Build history of the part. All positions in model axes, mm. A direction names the side the tool comes from. Round coordinates to 2 decimals unless told otherwise and drop trailing zeros. Loops run counter-clockwise (first coordinate to the right, second up) from the corner with the lowest first, then second, coordinate; pieces in that order, holes last. Notation, with made-up numbers: (54.25, -37.5) - (90.25, -37.5) arc R20 cw to (90.25, -16.5) - close; hole circle Ø11 at (72, 63.5). An arc over 180 degrees is marked (long way). Put each result on its own line as item: value. Start each with the question number.
from build123d import *

# Parameters (mm, degrees)
SKETCH1_W           = 10
SKETCH1_H           = 5
BOSS_EXTRUDE1_DEPTH = 5
SKETCH2_R           = 2.5
BOSS_EXTRUDE2_DEPTH = 5


with BuildPart() as part:
    # Sketch1 → Boss-Extrude1 (new body)
    with BuildSketch(Plane.XY):
        with Locations((-5, 2.5)):
            Rectangle(SKETCH1_W, SKETCH1_H)
    extrude(amount=BOSS_EXTRUDE1_DEPTH)

    # Sketch2 → Boss-Extrude2 (add)
    with BuildSketch(Plane.XY.offset(5)):
        with Locations(Location((-5, 2.5, 0), (0, 0, 270))):
            Circle(SKETCH2_R)
    extrude(amount=BOSS_EXTRUDE2_DEPTH)


solid = part.part
Item 1: Slice it at A-A (y = 2.5). Give the cut face in (x, z).
Item 2: Drill centre lines: probe 1 along Z at (x, y) = (-7.5, 3.75); probe 2 along X at (y, z) = (2.4, 5.25); probe 3 along X at (y, z) = (3.5, 6.5). Where is each one in solid material? Low to high. Write a range as [from, to].
Item 3: Slice it at C-C (y = 0.6). Give the cut face in (x, z).
Item 4: Slice it at B-B (z = 7.5). Give the cut face in (x, y), plus the area to 3 significant figures.
Item 5: Which spindle directions (+Z, -Z, +X, -X, +Y, -Y) get a long thin tool onto all of the face, cutting with end or side? Do faces 1 (the flat face through (-5, 3, 0)), 2 (the flat face through (-1, 3, 5)), 3 (the cylindrical face through (-3, 1, 7)). Say none if no direction does.
Computed values:
1. outline: (-10, 0) - (0, 0) - (0, 5) - (-2.5, 5) - (-2.5, 10) - (-7.5, 10) - (-7.5, 5) - (-10, 5) - close
2. probe 1: z = [0, 5]
2. probe 2: x = [-7.5, -2.5]
2. probe 3: x = [-7.29, -2.71]
3. outline: (-10, 0) - (0, 0) - (0, 5) - (-3.38, 5) - (-3.38, 10) - (-6.62, 10) - (-6.62, 5) - (-10, 5) - close
4. outline: circle Ø5 at (-5, 2.5)
4. area: 19.6 mm^2
5. face 1: -Z, +X, -X, +Y, -Y
5. face 2: +Z, +X
5. face 3: +Z
